Can you work these out from the model? Positions are in its coordinate system, mm. A direction names the side the tool comes from. Give positions to 0.01 mm unless a question says otherwise; leave off trailing zeros. Loops run counter-clockwise (first coordinate to the right, second up) from the corner with the lowest first, then second, coordinate; pieces in that order, holes last. Notation, with made-up numbers: (-8, 53) -> (50, 53) arc R30 cw to (50, 81) -> close; hole circle Ø11 at (77.25, 81.25). An arc over 180 degrees is marked (long way). Use CSV: the item, a comma, the result in double quotes.
from build123d import *

# Parameters (mm, degrees)
EXTRUDE1_DEPTH = 444.5
SKETCH2_R      = 4.826
SKETCH2_R_2    = 1.5875
EXTRUDE2_DEPTH = 25
SKETCH3_R      = 3.175
EXTRUDE3_DEPTH = 35


with BuildPart() as part:
    # Sketch1 → Extrude1 (new body, symmetric)
    with BuildSketch(Plane(origin=(0, 0, 0), x_dir=(1, 0, 0), z_dir=(0, 1, 0))):
        with BuildLine():
            Line((-12.7, 0), (-12.7, 22.225))
            ThreePointArc((-12.7, 22.225), (-11.77006403, 24.47006403), (-9.525, 25.4))
            Line((-9.525, 25.4), (9.525, 25.4))
            ThreePointArc((9.525, 25.4), (11.77006403, 24.47006403), (12.7, 22.225))
            Line((12.7, 22.225), (12.7, 0))
            Line((12.7, 0), (15.875, 0))
            Line((15.875, 0), (15.875, 22.225))
            ThreePointArc((15.875, 22.225), (14.015128061, 26.715128061), (9.525, 28.575))
            Line((9.525, 28.575), (-9.525, 28.575))
            ThreePointArc((-9.525, 28.575), (-14.015128061, 26.715128061), (-15.875, 22.225))
            Line((-15.875, 22.225), (-15.875, 0))
            Line((-15.875, 0), (-12.7, 0))
        make_face()
    extrude(amount=EXTRUDE1_DEPTH, both=True)

    # Sketch2 → Extrude2 (cut)
    with BuildSketch(Plane(origin=(0, 0, -28.575), x_dir=(-1, 0, 0), z_dir=(0, 0, -1))):
        with Locations((1.905, 361.95)):
            Circle(SKETCH2_R)
        with Locations((1.905, 336.55)):
            Circle(SKETCH2_R)
        with Locations((1.905, 107.95)):
            Circle(SKETCH2_R)
        with Locations((1.905, 82.55)):
            Circle(SKETCH2_R)
        with Locations((-1.905, 0)):
            Circle(SKETCH2_R)
        with Locations((1.905, -361.95)):
            Circle(SKETCH2_R)
        with Locations((1.905, -336.55)):
            Circle(SKETCH2_R)
        with Locations((1.905, -82.55)):
            Circle(SKETCH2_R)
        with Locations((1.905, -107.95)):
            Circle(SKETCH2_R)
        with Locations((0, -241.3)):
            Circle(SKETCH2_R_2)
    extrude(amount=-EXTRUDE2_DEPTH, mode=Mode.SUBTRACT)

    # Sketch3 → Extrude3 (cut)
    with BuildSketch(Plane(origin=(15.875, 0, 0), x_dir=(0, 0, -1), z_dir=(1, 0, 0))):
        with Locations((12.7, 431.8)):
            Circle(SKETCH3_R)
        with Locations((12.7, 406.4)):
            Circle(SKETCH3_R)
        with Locations((12.7, 381)):
            Circle(SKETCH3_R)
        with Locations((12.7, 355.6)):
            Circle(SKETCH3_R)
        with Locations((12.7, 330.2)):
            Circle(SKETCH3_R)
        with Locations((12.7, 304.8)):
            Circle(SKETCH3_R)
        with Locations((12.7, 279.4)):
            Circle(SKETCH3_R)
        with Locations((12.7, 254)):
            Circle(SKETCH3_R)
        with Locations((12.7, 228.6)):
            Circle(SKETCH3_R)
        with Locations((12.7, 203.2)):
            Circle(SKETCH3_R)
        with Locations((12.7, 177.8)):
            Circle(SKETCH3_R)
        with Locations((12.7, 152.4)):
            Circle(SKETCH3_R)
        with Locations((12.7, 127)):
            Circle(SKETCH3_R)
        with Locations((12.7, 101.6)):
            Circle(SKETCH3_R)
        with Locations((12.7, 76.2)):
            Circle(SKETCH3_R)
        with Locations((12.7, 50.8)):
            Circle(SKETCH3_R)
        with Locations((12.7, 25.4)):
            Circle(SKETCH3_R)
        with Locations((12.7, 0)):
            Circle(SKETCH3_R)
        with Locations((12.7, -25.4)):
            Circle(SKETCH3_R)
        with Locations((12.7, -50.8)):
            Circle(SKETCH3_R)
        with Locations((12.7, -76.2)):
            Circle(SKETCH3_R)
        with Locations((12.7, -101.6)):
            Circle(SKETCH3_R)
        with Locations((12.7, -127)):
            Circle(SKETCH3_R)
        with Locations((12.7, -152.4)):
            Circle(SKETCH3_R)
        with Locations((12.7, -177.8)):
            Circle(SKETCH3_R)
        with Locations((12.7, -203.2)):
            Circle(SKETCH3_R)
        with Locations((12.7, -228.6)):
            Circle(SKETCH3_R)
        with Locations((12.7, -254)):
            Circle(SKETCH3_R)
        with Locations((12.7, -279.4)):
            Circle(SKETCH3_R)
        with Locations((12.7, -304.8)):
            Circle(SKETCH3_R)
        with Locations((12.7, -330.2)):
            Circle(SKETCH3_R)
        with Locations((12.7, -355.6)):
            Circle(SKETCH3_R)
        with Locations((12.7, -381)):
            Circle(SKETCH3_R)
        with Locations((12.7, -406.4)):
            Circle(SKETCH3_R)
        with Locations((12.7, -431.8)):
            Circle(SKETCH3_R)
    extrude(amount=-EXTRUDE3_DEPTH, mode=Mode.SUBTRACT)


solid = part.part
(1) Which directions (+Z, -Z, +X, -X, +Y, -Y) give clear straight access to the entire face, cutting with the end or side of a thin tool? Please do faces 1 (the face through (0, 6, -28.575)), 2 (the face through (0, 6, -25.4)).
Answer sheet:
face 1,"-Z, +X, -X, +Y, -Y"
face 2,"+Z, +Y, -Y"
(2) Will these pins go through, and if not, where does the flat tip stop? pin 1 Ø2 at (x, y) = (-11, -315.5) entering from +Z; pin 2 Ø11 at (x, y) = (-1.905, -107.95) entering from +Z.
Answer sheet:
pin 1,"stops at z = -24.21"
pin 2,"stops at z = -25.4"
(3) If I drill on L1, parallel to X at y = 384, z = -21 (3 decimals); L2, parallel to X at y = 138.5, z = -24; L3, parallel to Z at x = 1.5, y = 268 (3 decimals), over which ranges is the centre line in solid material (lowest first)? Write a range as from..to.
Answer sheet:
L1,"x = -15.875..-12.7, 12.7..15.875"
L2,"x = -15.62..-12.16, 12.16..15.62"
L3,"z = -28.575..-25.4"
(4) We'd pull the mould along X, two halves only. Please class faces 3 (the face through (-15.875, 6, -11)), 4 (the face through (15.875, 6, -11)), 5 (the face through (0, -444.5, -26)), 6 (the face through (12.7, 6, -11)): released by +X, released by -X, zero draft, split by the parting line, or undercut.
Answer sheet:
face 3,"released by -X"
face 4,"released by +X"
face 5,"zero draft"
face 6,"undercut"
(5) If we section it at A-A, the plane y = 240.5: Write out the boundary of the cut face in (x, z) (3 decimals).
Answer sheet:
outline,"(-15.875, -22.225) arc R6.35 ccw to (-9.525, -28.575) -> (9.525, -28.575) arc R6.35 ccw to (15.875, -22.225) -> (15.875, 0) -> (12.7, 0) -> (12.7, -22.225) arc R3.175 cw to (9.525, -25.4) -> (-9.525, -25.4) arc R3.175 cw to (-12.7, -22.225) -> (-12.7, 0) -> (-15.875, 0) -> close"
